Autodesk Inventor part; units mm, degrees
ref_plane "YZ Plane" through (0, 0, 0) normal (1, 0, 0) x (0, 1, 0)
ref_plane "XZ Plane" through (0, 0, 0) normal (0, 1, 0) x (-1, 0, 0)
ref_plane "XY Plane" through (0, 0, 0) normal (0, 0, 1) x (1, 0, 0)
sketch "Sketch1" plane through (0, 0, 0) normal (0, 1, 0) x (-1, 0, 0)
  line L0 (0, 0) -> (60, 0)
  line L1 (60, 0) -> (60, -100)
  line L2 (60, -100) -> (0, -100)
  line L3 (0, -100) -> (0, 0)
  dimension "d0" = 60
  dimension "d1" = 100
extrude "Extrusion1" add sketch "Sketch1" along normal blind 10
sketch "Sketch2" plane through (0, 10, 0) normal (0, 1, 0) x (1, 0, 0)
  circle A0 centre (-52.5, 60.625) radius 1
  line L0 (0, 100) -> (-60, 100)
  line L1 (-60, 100) -> (-60, 0)
  point P0 (0, 0)
  dimension "d4" = 2
  dimension "d5" = 39.375
  dimension "d6" = 7.5
extrude "Extrusion2" cut sketch "Sketch2" against normal blind 10
sketch "Sketch3" plane through (0, 10, 0) normal (0, 1, 0) x (1, 0, 0)
  circle A0 centre (-52.5, 36.625) radius 1
  circle A1 centre (-52.5, 60.625) radius 1
  point P0 (0, 0)
  dimension "d9" = 2
  dimension "d10" = 24
  dimension "d11" = 0
extrude "Extrusion3" cut sketch "Sketch3" against normal blind 10 contours A0
sketch "Sketch4" plane through (0, 10, 0) normal (0, 1, 0) x (1, 0, 0)
  circle A0 centre (-52.5, 92.5) radius 1
  line L0 (0, 100) -> (-60, 100)
  line L1 (-60, 100) -> (-60, 0)
  point P0 (0, 0)
  dimension "d14" = 2
  dimension "d15" = 7.5
  dimension "d16" = 7.5
extrude "Extrusion4" cut sketch "Sketch4" against normal blind 10
properties part number "temp back plate"
Geometry check sheet. Reference: the model listing, model coordinates, mm. Round coordinates to 2 decimals unless told otherwise and drop trailing zeros. Loops run counter-clockwise (first coordinate to the right, second up) from the corner with the lowest first, then second, coordinate; pieces in that order, holes last.
Item 1: Cross-section at B-B on x = -52.5. Record the boundary of the cut face in (y, z) (3 decimals).
Item 2: Thickness scan on line 1 (Z direction, x = -52.5, y = 7) (3 decimals); line 2 (X direction, y = 8.25, z = -92.5); line 3 (X direction, y = 2.75, z = -37). Record the ranges inside material, lowest first.
Item 3: Mould release check, pull along X, two halves, no side actions. Record for faces 1 (the cylindrical face through (-51.962, 5.07, -61.468)), 2 (the flat face through (-30, 10, -49)), 3 (the flat face through (-60, 5, -49)): pulls with the +X half, pulls with the -X half, needs draft (parallel to the pull), parting line crosses it, or undercut.
Item 4: Gauge pin test, flat end, axial feed: pin 1 (1.6 mm diameter, centred on x = -52.5, z = -92.5, fed in from -Y). Record the tip position at first contact, or that the pin passes through.
Item 5: Cross-section at A-A on z = -92.5. Record the boundary of the cut face in (x, y).
Answer sheet:
1. outline: (0, -100) - (10, -100) - (10, -93.5) - (0, -93.5) - close; (0, -91.5) - (10, -91.5) - (10, -61.625) - (0, -61.625) - close; (0, -59.625) - (10, -59.625) - (10, -37.625) - (0, -37.625) - close; (0, -35.625) - (10, -35.625) - (10, 0) - (0, 0) - close
2. line 1: z = -100 to -93.5, -91.5 to -61.625, -59.625 to -37.625, -35.625 to 0
2. line 2: x = -60 to -53.5, -51.5 to 0
2. line 3: x = -60 to -53.43, -51.57 to 0
3. face 1: undercut
3. face 2: needs draft
3. face 3: pulls with the -X half
4. pin 1: passes through
5. outline: (-60, 0) - (-53.5, 0) - (-53.5, 10) - (-60, 10) - close; (-51.5, 0) - (0, 0) - (0, 10) - (-51.5, 10) - close
